from build123d import *

# Parameters (mm, degrees)
SKETCH1_W                      = 3.1
SKETCH1_H                      = 10
BOSS_EXTRUDE1_DEPTH            = 3
F_6_1_6_1_DIAMETER_HOLE1_D     = 6.1
F_6_1_6_1_DIAMETER_HOLE1_DEPTH = 10
F_6_1_6_1_DIAMETER_HOLE1_TIP   = 1.832624888


with BuildPart() as part:
    # Sketch1 → Boss-Extrude1 (new body)
    with BuildSketch(Plane(origin=(0, 0, 0), x_dir=(1, 0, 0), z_dir=(0, 1, 0))):
        with BuildLine():
            Line((-14.890188717, 16.254064822), (-12.620010218, 42.260882944))
            ThreePointArc((-12.620010218, 42.260882944), (-11.658361887, 44.211633879), (-9.631375063, 45))
            Line((-9.631375063, 45), (9.631375063, 45))
            ThreePointArc((9.631375063, 45), (11.658361887, 44.211633879), (12.620010218, 42.260882944))
            Line((12.620010218, 42.260882944), (14.890188717, 16.254064822))
            ThreePointArc((14.890188717, 16.254064822), (15.323846122, 15.323846122), (16.254064822, 14.890188717))
            Line((16.254064822, 14.890188717), (42.260882944, 12.620010218))
            ThreePointArc((42.260882944, 12.620010218), (44.211633879, 11.658361887), (45, 9.631375063))
            Line((45, 9.631375063), (45, -9.631375063))
            ThreePointArc((45, -9.631375063), (44.211633879, -11.658361887), (42.260882944, -12.620010218))
            Line((42.260882944, -12.620010218), (16.254064822, -14.890188717))
            ThreePointArc((16.254064822, -14.890188717), (15.323846122, -15.323846122), (14.890188717, -16.254064822))
            Line((14.890188717, -16.254064822), (12.620010218, -42.260882944))
            ThreePointArc((12.620010218, -42.260882944), (11.658361887, -44.211633879), (9.631375063, -45))
            Line((9.631375063, -45), (-9.631375063, -45))
            ThreePointArc((-9.631375063, -45), (-11.658361887, -44.211633879), (-12.620010218, -42.260882944))
            Line((-12.620010218, -42.260882944), (-14.890188717, -16.254064822))
            ThreePointArc((-14.890188717, -16.254064822), (-15.323846122, -15.323846122), (-16.254064822, -14.890188717))
            Line((-16.254064822, -14.890188717), (-42.260882944, -12.620010218))
            ThreePointArc((-42.260882944, -12.620010218), (-44.211633879, -11.658361887), (-45, -9.631375063))
            Line((-45, -9.631375063), (-45, 9.631375063))
            ThreePointArc((-45, 9.631375063), (-44.211633879, 11.658361887), (-42.260882944, 12.620010218))
            Line((-42.260882944, 12.620010218), (-16.254064822, 14.890188717))
            ThreePointArc((-16.254064822, 14.890188717), (-15.323846122, 15.323846122), (-14.890188717, 16.254064822))
        make_face()
        with Locations((-4.1, 10)):
            Rectangle(SKETCH1_W, SKETCH1_H, mode=Mode.SUBTRACT)
        with Locations((4.1, 10)):
            Rectangle(SKETCH1_W, SKETCH1_H, mode=Mode.SUBTRACT)
        with Locations((4.1, -10)):
            Rectangle(SKETCH1_W, SKETCH1_H, mode=Mode.SUBTRACT)
        with Locations((-4.1, -10)):
            Rectangle(SKETCH1_W, SKETCH1_H, mode=Mode.SUBTRACT)
    extrude(amount=BOSS_EXTRUDE1_DEPTH)

    # Ø6.1 (6.1) Diameter Hole1
    with Locations(Plane(origin=(0, 3, 0), x_dir=(1, 0, 0), z_dir=(0, 1, 0))):
        with Locations((0, -30), (30, 0), (0, 30), (-30, 0)):
            Hole(F_6_1_6_1_DIAMETER_HOLE1_D / 2, depth=F_6_1_6_1_DIAMETER_HOLE1_DEPTH)
            with Locations((0, 0, -(F_6_1_6_1_DIAMETER_HOLE1_DEPTH + F_6_1_6_1_DIAMETER_HOLE1_TIP / 2))):  # 118° drill point
                Cone(0, F_6_1_6_1_DIAMETER_HOLE1_D / 2, F_6_1_6_1_DIAMETER_HOLE1_TIP, mode=Mode.SUBTRACT)


solid = part.part
Source: CAD feature listing. Evaluate the final solid. Frame: model axes, mm. A direction names the side the tool comes from. Coordinates: 2 decimals unless noted, no trailing zeros. Order: outer loops, then holes, each group sorted by start corner. A loop starts at its lowest first (then second) coordinate and runs counter-clockwise, first axis right, second up.
Item 1: First-contact query: P1, Ø0.9, axis at y = 2, z = -11, coming from the +X side; P2, Ø1, axis at y = 2, z = 33.5, coming from the -X side; P3, Ø1, axis at x = -34.5, y = 1, coming from the -Z side. Flat tips, straight axial feed; report the tip coordinate or a pass-through.
Output values:
P1: stops at x = 44.86
P2: stops at x = -13.43
P3: stops at z = -13.34
Item 2: Set-up query: faces 1 (the face through (0, 1, 45)), 2 (the face through (-2.55, 1, -10)). Return all of +Z, -Z, +X, -X, +Y, -Y with unobstructed straight access to the full face (end or side cutting, diameter ignored); none if empty.
Output values:
face 1: +Z, +X, -X, +Y, -Y
face 2: +Y, -Y
Item 3: Cut plane C-C (x = -30). Return loops of the section in (y, z), plus the area to 3 significant figures.
Output values:
outline: (0, -13.69) - (3, -13.69) - (3, -3.05) - (0, -3.05) - close; (0, 3.05) - (3, 3.05) - (3, 13.69) - (0, 13.69) - close
area: 63.8 mm2
Item 4: Cut plane A-A (z = 0). Return loops of the section in (x, y).
Output values:
outline: (-45, 0) - (-33.05, 0) - (-33.05, 3) - (-45, 3) - close; (-26.95, 0) - (26.95, 0) - (26.95, 3) - (-26.95, 3) - close; (33.05, 0) - (45, 0) - (45, 3) - (33.05, 3) - close
Item 5: Pull-direction query (X, two-part tool) for faces 3 (the face through (-11.68, 1.48, -44.19)), 4 (the face through (1, 3, -1)), 5 (the face through (5.65, 1, 10)); classes: pulls with the +X half, pulls with the -X half, needs draft (parallel to the pull), parting line crosses it, or undercut.
Output values:
face 3: pulls with the -X half
face 4: needs draft
face 5: undercut
Item 6: Material intervals for line 1 (Z direction, x = 0, y = 0.8); line 2 (X direction, y = 1.75, z = 30); line 3 (X direction, y = 1.6, z = -1), sorted ascending.
Output values:
line 1: z = -45 to -33.05, -26.95 to 26.95, 33.05 to 45
line 2: x = -13.69 to -3.05, 3.05 to 13.69
line 3: x = -45 to -32.88, -27.12 to 27.12, 32.88 to 45
Item 7: Cut plane D-D (z = -30). Return loops of the section in (x, y).
Output values:
outline: (-13.69, 0) - (-3.05, 0) - (-3.05, 3) - (-13.69, 3) - close; (3.05, 0) - (13.69, 0) - (13.69, 3) - (3.05, 3) - close
Item 8: Cut plane B-B (x = 0). Return loops of the section in (y, z), plus the area to 3 significant figures.
Output values:
outline: (0, -45) - (3, -45) - (3, -33.05) - (0, -33.05) - close; (0, -26.95) - (3, -26.95) - (3, 26.95) - (0, 26.95) - close; (0, 33.05) - (3, 33.05) - (3, 45) - (0, 45) - close
area: 233 mm2
